Model file for the job. Use its own axes, mm. Face numbers are marked on the shaded views. A direction names the side the tool comes from. Coordinates: 2 decimals unless noted, no trailing zeros. Loops run counter-clockwise (first coordinate to the right, second up) from the corner with the lowest first, then second, coordinate; pieces in that order, holes last. Notation, with made-up numbers: (-26, -34.75) -> (25, -34.75) arc R25 cw to (25, -8.75) -> close; hole circle Ø4 at (67.5, -24.75). An arc over 180 degrees is marked (long way). Use one line per item in the form item = value.
```python
from build123d import *

# Parameters (mm, degrees)
CROQUIS1_W               = 42.5
CROQUIS1_H               = 42.5
SALIENTE_EXTRUIR1_DEPTH  = 5
CROQUIS6_W               = 5
CROQUIS6_H               = 42.5
SALIENTE_EXTRUIR2_DEPTH  = 4
CROQUIS7_W               = 4
CROQUIS7_H               = 42.5
SALIENTE_EXTRUIR3_DEPTH  = 42.5
CROQUIS8_R               = 11.25
CROQUIS8_R_2             = 1.6
CORTAR_EXTRUIR2_DEPTH    = 4
CROQUIS10_W              = 4
CROQUIS10_H              = 3.5
SALIENTE_EXTRUIR4_DEPTH  = 12
CROQUIS11_W              = 12
CROQUIS11_H              = 3.5
SALIENTE_EXTRUIR5_DEPTH  = 22
CROQUIS12_R              = 1.6
CORTAR_EXTRUIR4_DEPTH    = 3.5
REDONDEO1_R              = 5
REDONDEO2_R              = 5
REDONDEO3_R              = 4
CORTAR_EXTRUIR5_DEPTH    = 0.7
CROQUIS14_W              = 5
CROQUIS14_H              = 42.5
SALIENTE_EXTRUIR6_DEPTH  = 18
CROQUIS15_R              = 1.75
CORTAR_EXTRUIR6_DEPTH    = 5
CROQUIS16_R              = 2.8
CORTAR_EXTRUIR7_DEPTH    = 3.5
CROQUIS17_R              = 2.8
CORTAR_EXTRUIR8_DEPTH    = 3.5
REDONDEO5_R              = 5
CROQUIS18_R              = 1.6
SALIENTE_EXTRUIR8_DEPTH  = 2
CROQUIS19_R              = 1.6
CORTAR_EXTRUIR9_DEPTH    = 2
REDONDEO7_R              = 3
REDONDEO8_R              = 3
SALIENTE_EXTRUIR9_DEPTH  = 2
SALIENTE_EXTRUIR10_DEPTH = 2
CROQUIS22_W              = 26.97020456
CROQUIS22_H              = 2
CORTAR_EXTRUIR10_DEPTH   = 5
CROQUIS23_W              = 1.770204561
CROQUIS23_H              = 2
CORTAR_EXTRUIR11_DEPTH   = 5
REDONDEO9_R              = 3


with BuildPart() as part:
    # Croquis1 → Saliente-Extruir1 (new body)
    with BuildSketch(Plane(origin=(0, 0, 0), x_dir=(0, 0, -1), z_dir=(1, 0, 0))):
        with Locations((-2.329734219, -7.130398671)):
            Rectangle(CROQUIS1_W, CROQUIS1_H)
    extrude(amount=-SALIENTE_EXTRUIR1_DEPTH)

    # Croquis6 → Saliente-Extruir2 (add)
    with BuildSketch(Plane(origin=(0, 0, -18.920265781), x_dir=(-1, 0, 0), z_dir=(0, 0, -1))):
        with Locations((2.5, -7.130398671)):
            Rectangle(CROQUIS6_W, CROQUIS6_H)
    extrude(amount=SALIENTE_EXTRUIR2_DEPTH)

    # Croquis7 → Saliente-Extruir3 (add)
    with BuildSketch(Plane.ZY.offset(5)):
        with Locations((-20.920265781, -7.130398671)):
            Rectangle(CROQUIS7_W, CROQUIS7_H)
    extrude(amount=SALIENTE_EXTRUIR3_DEPTH)

    # Croquis8 → Cortar-Extruir2 (cut)
    with BuildSketch(Plane.XY.offset(-18.920265781)):
        with Locations((-26.25, -7.130398671)):
            Circle(CROQUIS8_R)
        with Locations((-41.75, 8.369601329)):
            Circle(CROQUIS8_R_2)
        with Locations((-10.75, 8.369601329)):
            Circle(CROQUIS8_R_2)
        with Locations((-10.75, -22.630398671)):
            Circle(CROQUIS8_R_2)
        with Locations((-41.75, -22.630398671)):
            Circle(CROQUIS8_R_2)
    extrude(amount=-CORTAR_EXTRUIR2_DEPTH, mode=Mode.SUBTRACT)

    # Croquis10 → Saliente-Extruir4 (add)
    with BuildSketch(Plane.ZY.offset(47.5)):
        with Locations((-20.920265781, -6.630398671)):
            Rectangle(CROQUIS10_W, CROQUIS10_H)
    extrude(amount=SALIENTE_EXTRUIR4_DEPTH)

    # Croquis11 → Saliente-Extruir5 (add)
    with BuildSketch(Plane.XY.offset(-18.920265781)):
        with Locations((-53.5, -6.630398671)):
            Rectangle(CROQUIS11_W, CROQUIS11_H)
    extrude(amount=SALIENTE_EXTRUIR5_DEPTH)

    # Croquis12 → Cortar-Extruir4 (cut)
    with BuildSketch(Plane(origin=(0, -4.880398671, 0), x_dir=(1, 0, 0), z_dir=(0, 1, 0))):
        with Locations(Location((-53.5, 18.920265781, 0), (0, 0, 270))):
            Circle(CROQUIS12_R)
        with Locations(Location((-53.5, 0.920265781, 0), (0, 0, 270))):
            Circle(CROQUIS12_R)
    extrude(amount=-CORTAR_EXTRUIR4_DEPTH, mode=Mode.SUBTRACT)

    # Redondeo1
    redondeo1_edges = [part.edges().sort_by_distance(p)[0] for p in [
        (-2.5, -28.380398671, 23.579734219),
        (-2.5, 14.119601329, 23.579734219),
    ]]
    fillet(redondeo1_edges, radius=REDONDEO1_R)

    # Redondeo2
    redondeo2_edges = [part.edges().sort_by_distance(p)[0] for p in [
        (-47.5, -28.380398671, -20.920265781),
        (-47.5, 14.119601329, -20.920265781),
    ]]
    fillet(redondeo2_edges, radius=REDONDEO2_R)

    # Redondeo3
    redondeo3_edges = [part.edges().sort_by_distance(p)[0] for p in [
        (-59.5, -6.630398671, -22.920265781),
        (-59.5, -6.630398671, 3.079734219),
        (-47.5, -6.630398671, 3.079734219),
    ]]
    fillet(redondeo3_edges, radius=REDONDEO3_R)

    # Croquis13 → Cortar-Extruir5 (cut)
    with BuildSketch(Plane.XY.offset(-18.920265781)):
        with BuildLine():
            Line((-47.5, -8.380398671), (-47.5, -23.380398671))
            ThreePointArc((-47.5, -23.380398671), (-46.035533906, -26.915932577), (-42.5, -28.380398671))
            Line((-42.5, -28.380398671), (-5, -28.380398671))
            Line((-5, -28.380398671), (-5, 14.119601329))
            Line((-5, 14.119601329), (-42.5, 14.119601329))
            ThreePointArc((-42.5, 14.119601329), (-46.035533906, 12.655135235), (-47.5, 9.119601329))
            Line((-47.5, 9.119601329), (-47.5, -4.880398671))
            Line((-47.5, -4.880398671), (-47.5, -8.380398671))
        make_face()
    extrude(amount=-CORTAR_EXTRUIR5_DEPTH, mode=Mode.SUBTRACT)

    # Croquis14 → Saliente-Extruir6 (add)
    with BuildSketch(Plane(origin=(0, 0, -22.920265781), x_dir=(-1, 0, 0), z_dir=(0, 0, -1))):
        with Locations((2.5, -7.130398671)):
            Rectangle(CROQUIS14_W, CROQUIS14_H)
    extrude(amount=SALIENTE_EXTRUIR6_DEPTH)

    # Croquis15 → Cortar-Extruir6 (cut)
    with BuildSketch(Plane(origin=(0, 0, 0), x_dir=(0, 0, -1), z_dir=(1, 0, 0))):
        with Locations((9.920265781, 4.369601329)):
            Circle(CROQUIS15_R)
        with Locations((32.920265781, 4.369601329)):
            Circle(CROQUIS15_R)
        with Locations((32.920265781, -18.630398671)):
            Circle(CROQUIS15_R)
        with Locations((9.920265781, -18.630398671)):
            Circle(CROQUIS15_R)
    extrude(amount=-CORTAR_EXTRUIR6_DEPTH, mode=Mode.SUBTRACT)

    # Croquis16 → Cortar-Extruir7 (cut)
    with BuildSketch(Plane.ZY.offset(5)):
        with Locations((-9.920265781, 4.369601329)):
            Circle(CROQUIS16_R)
        with Locations((-9.920265781, -18.630398671)):
            Circle(CROQUIS16_R)
    extrude(amount=-CORTAR_EXTRUIR7_DEPTH, mode=Mode.SUBTRACT)

    # Croquis17 → Cortar-Extruir8 (cut)
    with BuildSketch(Plane.ZY.offset(5)):
        with Locations(Location((-32.920265781, 4.369601329, 0), (0, 0, 270))):
            Circle(CROQUIS17_R)
        with Locations(Location((-32.920265781, -18.630398671, 0), (0, 0, 270))):
            Circle(CROQUIS17_R)
    extrude(amount=-CORTAR_EXTRUIR8_DEPTH, mode=Mode.SUBTRACT)

    # Redondeo5
    redondeo5_edges = [part.edges().sort_by_distance(p)[0] for p in [
        (-2.5, -28.380398671, -40.920265781),
        (-2.5, 14.119601329, -40.920265781),
    ]]
    fillet(redondeo5_edges, radius=REDONDEO5_R)

    # Croquis18 → Saliente-Extruir8 (add)
    with BuildSketch(Plane.XZ.offset(8.380398671)):
        with BuildLine():
            Line((-59.5, -0.920265781), (-59.5, -18.920265781))
            ThreePointArc((-59.5, -18.920265781), (-58.328427125, -21.748692905), (-55.5, -22.920265781))
            Line((-55.5, -22.920265781), (-47.5, -22.920265781))
            Line((-47.5, -22.920265781), (-47.5, -19.620265781))
            Line((-47.5, -19.620265781), (-47.5, -0.920265781))
            ThreePointArc((-47.5, -0.920265781), (-48.671572875, 1.908161344), (-51.5, 3.079734219))
            Line((-51.5, 3.079734219), (-55.5, 3.079734219))
            ThreePointArc((-55.5, 3.079734219), (-58.328427125, 1.908161344), (-59.5, -0.920265781))
        make_face()
        with Locations(Location((-53.5, -0.920265781, 0), (0, 0, 90))):
            Circle(CROQUIS18_R, mode=Mode.SUBTRACT)
        with Locations(Location((-53.5, -18.920265781, 0), (0, 0, 90))):
            Circle(CROQUIS18_R, mode=Mode.SUBTRACT)
    extrude(amount=SALIENTE_EXTRUIR8_DEPTH)

    # Croquis19 → Cortar-Extruir9 (cut)
    with BuildSketch(Plane(origin=(0, -4.880398671, 0), x_dir=(1, 0, 0), z_dir=(0, 1, 0))):
        with BuildLine():
            Line((-51.5, -3.079734219), (-55.5, -3.079734219))
            ThreePointArc((-55.5, -3.079734219), (-58.328427125, -1.908161344), (-59.5, 0.920265781))
            Line((-59.5, 0.920265781), (-59.5, 18.920265781))
            ThreePointArc((-59.5, 18.920265781), (-58.328427125, 21.748692905), (-55.5, 22.920265781))
            Line((-55.5, 22.920265781), (-47.5, 22.920265781))
            Line((-47.5, 22.920265781), (-47.5, 19.620265781))
            Line((-47.5, 19.620265781), (-47.5, 0.920265781))
            ThreePointArc((-47.5, 0.920265781), (-48.671572875, -1.908161344), (-51.5, -3.079734219))
        make_face()
        with Locations(Location((-53.5, 18.920265781, 0), (0, 0, 270))):
            Circle(CROQUIS19_R, mode=Mode.SUBTRACT)
        with Locations(Location((-53.5, 0.920265781, 0), (0, 0, 270))):
            Circle(CROQUIS19_R, mode=Mode.SUBTRACT)
    extrude(amount=-CORTAR_EXTRUIR9_DEPTH, mode=Mode.SUBTRACT)

    # Redondeo7
    redondeo7_edges = [part.edges().sort_by_distance(p)[0] for p in [
        (-47.5, -6.880398671, -21.270265781),
    ]]
    fillet(redondeo7_edges, radius=REDONDEO7_R)

    # Redondeo8
    redondeo8_edges = [part.edges().sort_by_distance(p)[0] for p in [
        (-47.5, -10.380398671, -21.270265781),
    ]]
    fillet(redondeo8_edges, radius=REDONDEO8_R)

    # Croquis20 → Saliente-Extruir9 (add)
    with BuildSketch(Plane.XZ.offset(28.380398671)):
        Polygon((-5, -22.920265781), (-5, -35.920265781), (0, -35.920265781), (0, 18.579734219), (-5, 18.579734219), (-5, -19.620265781), (-42.5, -19.620265781), (-42.5, -22.920265781), align=None)
    extrude(amount=SALIENTE_EXTRUIR9_DEPTH)

    # Croquis21 → Saliente-Extruir10 (add)
    with BuildSketch(Plane.XZ.offset(30.380398671)):
        with BuildLine():
            Line((-16.22979544, -19.620265781), (-5, -19.620265781))
            Line((-5, -19.620265781), (-5, -8.390470341))
            ThreePointArc((-5, -8.390470341), (-8.771291942, -15.848973839), (-16.22979544, -19.620265781))
        make_face()
        with BuildLine():
            ThreePointArc((-16.22979544, -22.920265781), (-8.525539397, -26.445805177), (-5, -34.15006122))
            Line((-5, -34.15006122), (-5, -22.920265781))
            Line((-5, -22.920265781), (-16.22979544, -22.920265781))
        make_face()
    extrude(amount=-SALIENTE_EXTRUIR10_DEPTH)

    # Croquis22 → Cortar-Extruir10 (cut)
    with BuildSketch(Plane.ZY.offset(5)):
        with Locations((5.094631939, -29.380398671)):
            Rectangle(CROQUIS22_W, CROQUIS22_H)
    extrude(amount=-CORTAR_EXTRUIR10_DEPTH, mode=Mode.SUBTRACT)

    # Croquis23 → Cortar-Extruir11 (cut)
    with BuildSketch(Plane.ZY.offset(5)):
        with Locations((-35.035163501, -29.380398671)):
            Rectangle(CROQUIS23_W, CROQUIS23_H)
    extrude(amount=-CORTAR_EXTRUIR11_DEPTH, mode=Mode.SUBTRACT)

    # Redondeo9
    # the kernel refuses this fillet: 3 mm, written as the material it adds along each edge
    with BuildSketch(Plane(origin=(-5, -28.380398671, -34.15006122), x_dir=(0, -1, 0), z_dir=(1, 0, 0))) as redondeo9_piece_1:
        with BuildLine():
            CenterArc((2.926328174, 2.853404303), REDONDEO9_R, 187.781748717, 64.232765745)
            Line((-0.046044891, 2.447204399), (-0.343282198, 2.406584409))
            ThreePointArc((-0.343282198, 2.406584409), (-0.3, 1.77020456), (-0.3, 0))
            Line((-0.3, 0), (0, -0.3))
            ThreePointArc((0, -0.3), (1, -0.3), (1.907367183, -0.28534043))
            Line((1.907367183, -0.28534043), (2, 0))
        make_face()
    extrude(amount=5)
    with BuildSketch(Plane(origin=(-5, -28.380398671, -8.390470341), x_dir=(0, -1, 0), z_dir=(1, 0, 0))) as redondeo9_piece_2:
        with BuildLine():
            CenterArc((3, -2.828427125), REDONDEO9_R, 109.471220634, 70.528779366)
            Line((0, -2.828427125), (0, 0))
            Line((0, 0), (2, 0))
        make_face()
    extrude(amount=5)


solid = part.part
```
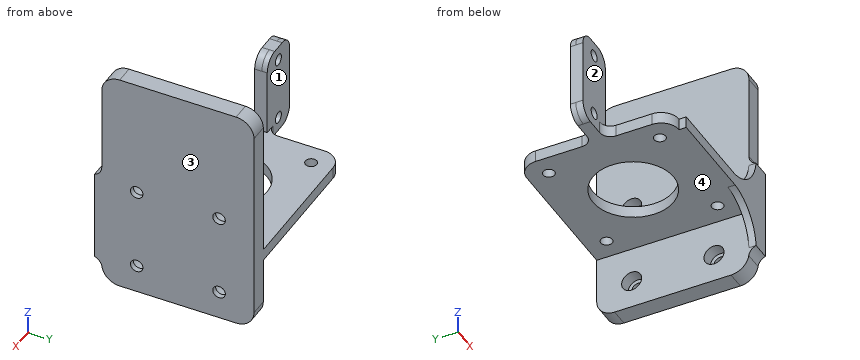
Q1. Band-saw the part on B-B, the plane x = -26.25. Write the cut outline in (y, z), and give its area (3 significant figures).
Result:
outline = (-30.38, -22.92) -> (-18.38, -22.92) -> (-18.38, -19.62) -> (-30.38, -19.62) -> close; (4.12, -22.92) -> (14.12, -22.92) -> (14.12, -19.62) -> (4.12, -19.62) -> close
area = 72.6 mm2
Q2. Band-saw the part on D-D, the plane z = 12. Write the cut outline in (x, y).
Result:
outline = (-5, -28.38) -> (0, -28.38) -> (0, 14.12) -> (-5, 14.12) -> close
Q3. Band-saw the part on A-A, the plane x = -53.5. Write the cut outline in (y, z).
Result:
outline = (-10.38, -22.92) -> (-6.88, -22.92) -> (-6.88, -20.52) -> (-10.38, -20.52) -> close; (-10.38, -17.32) -> (-6.88, -17.32) -> (-6.88, -2.52) -> (-10.38, -2.52) -> close; (-10.38, 0.68) -> (-6.88, 0.68) -> (-6.88, 3.08) -> (-10.38, 3.08) -> close
Q4. Band-saw the part on C-C, the plane y = -19.5. Write the cut outline in (x, z).
Result:
outline = (-47.5, -22.92) -> (-5, -22.92) -> (-5, -30.26) -> (-1.5, -30.26) -> (-1.5, -31.4) -> (0, -31.4) -> (0, -11.44) -> (-1.5, -11.44) -> (-1.5, -12.58) -> (-5, -12.58) -> (-5, -19.62) -> (-47.5, -19.62) -> close; (-5, -40.92) -> (0, -40.92) -> (0, -34.44) -> (-1.5, -34.44) -> (-1.5, -35.58) -> (-5, -35.58) -> close; (-5, -7.26) -> (-1.5, -7.26) -> (-1.5, -8.4) -> (0, -8.4) -> (0, 23.58) -> (-5, 23.58) -> close
Q5. Wall check: line 1 along Z through (x, y) = (-53.5, -8.55); line 2 along Y through (x, z) = (-10, -20); line 3 along Z through (x, y) = (-43, -25.5). Give the ranges that are in metal, low to high.
Result:
line_1 = -22.92 to -20.52, -17.32 to -2.52, 0.68 to 3.08
line_2 = -30.38 to -24.04, -21.22 to 6.96, 9.78 to 14.12
line_3 = -22.92 to -19.62
Q6. Which spindle directions (+Z, -Z, +X, -X, +Y, -Y) get a long thin tool onto all of the face, cutting with end or side? Do the marked faces 1, 2, 3 and 4. Say none if no direction does.
Result:
face_1 = +Z, -X, +Y
face_2 = +Z, -X, -Y
face_3 = +Z, -Z, +X, +Y, -Y
face_4 = -Z, -X, +Y
Q7. Pin check, flat tips, straight feed: pin 1 Ø4 at (x, z) = (-18, -19.5) entering from -Y; pin 2 Ø21.5 at (y, z) = (-6.5, 10.5) entering from -X; pin 3 Ø4.5 at (y, z) = (4.5, -34.5) entering from -X; pin 4 Ø4.5 at (y, z) = (-18.63, -32.92) entering from -X. Stop position of each tip, or through.
Result:
pin_1 = -30.38
pin_2 = -59.44
pin_3 = -5
pin_4 = -1.5
